CAD build for the part. Positions are in the model's coordinates, mm. Face numbers are marked on the shaded views. A direction names the side the tool comes from. Round coordinates to 2 decimals unless told otherwise and drop trailing zeros. Loops run counter-clockwise (first coordinate to the right, second up) from the corner with the lowest first, then second, coordinate; pieces in that order, holes last. Notation, with made-up numbers: M 41.25,-35.75 L 77.25,-35.75 A22 ccw 77.25,-10.75 Z; hole C 29,50 d2. An arc over 180 degrees is marked long. One line per item, written item: value. Start each with the question number.
from build123d import *

# Parameters (mm, degrees)
SKETCH2_R           = 5
BOSS_EXTRUDE1_DEPTH = 62.5
SKETCH3_R           = 8
BOSS_EXTRUDE2_DEPTH = 7.5
FILLET1_R           = 5
SKETCH4_R           = 10
BOSS_EXTRUDE3_DEPTH = 7.5
CHAMFER1_SIZE       = 2


# Some blends are built 0.0001 mm under size
with BuildPart() as part:
    # Sketch2 → Boss-Extrude1 (new, symmetric)
    with BuildSketch(Plane(origin=(0, 0, 0), x_dir=(0, 0, -1), z_dir=(1, 0, 0))):
        Circle(SKETCH2_R)
    extrude(amount=BOSS_EXTRUDE1_DEPTH, both=True)

    # Sketch3 → Boss-Extrude2 (add, symmetric)
    with BuildSketch(Plane(origin=(0, 0, 0), x_dir=(0, 0, -1), z_dir=(1, 0, 0))):
        Circle(SKETCH3_R)
    extrude(amount=BOSS_EXTRUDE2_DEPTH, both=True)

    # Fillet1
    # the kernel refuses this fillet: 5 mm, written as the material it adds along each edge
    with BuildSketch(Plane(origin=(-7.5, 0, 0), x_dir=(0, 0, -1), z_dir=(0, -1, 0))) as fillet1_piece_1:
        with BuildLine():
            CenterArc((10, -4.582575695), FILLET1_R, 113.578178478, 66.421821522)
            Line((8, 0), (7.96, 0.091651514))
            ThreePointArc((7.96, 0.091651514), (6.5, 0.1), (5, 0.1))
            Line((5, 0.1), (4.9, 0))
            Line((4.9, 0), (4.9, -4.582575695))
            Line((4.9, -4.582575695), (5, -4.582575695))
        make_face()
    revolve(axis=Axis((-7.5, 0, 0), (1, 0, 0)))
    with BuildSketch(Plane(origin=(7.5, 0, 0), x_dir=(0, 0, -1), z_dir=(0, -1, 0))) as fillet1_piece_2:
        with BuildLine():
            CenterArc((10, 4.582575695), FILLET1_R, 180, 66.421821522)
            Line((5, 4.582575695), (4.9, 4.582575695))
            Line((4.9, 4.582575695), (4.9, 0))
            Line((4.9, 0), (5, -0.1))
            ThreePointArc((5, -0.1), (6.5, -0.1), (7.96, -0.091651514))
            Line((7.96, -0.091651514), (8, 0))
        make_face()
    revolve(axis=Axis((7.5, 0, 0), (1, 0, 0)))

    # Sketch4 → Boss-Extrude3 (add, symmetric)
    with BuildSketch(Plane(origin=(0, 0, 0), x_dir=(0, 0, -1), z_dir=(1, 0, 0))):
        Circle(SKETCH4_R)
    extrude(amount=BOSS_EXTRUDE3_DEPTH, both=True)

    # Chamfer1
    chamfer1_edges = [part.edges().sort_by_distance(p)[0] for p in [
        (-7.5, 0, 10),
        (7.5, 0, 10),
    ]]
    chamfer(chamfer1_edges, length=CHAMFER1_SIZE - 0.0001)  # a hair under: the kernel refuses the full size


solid = part.part
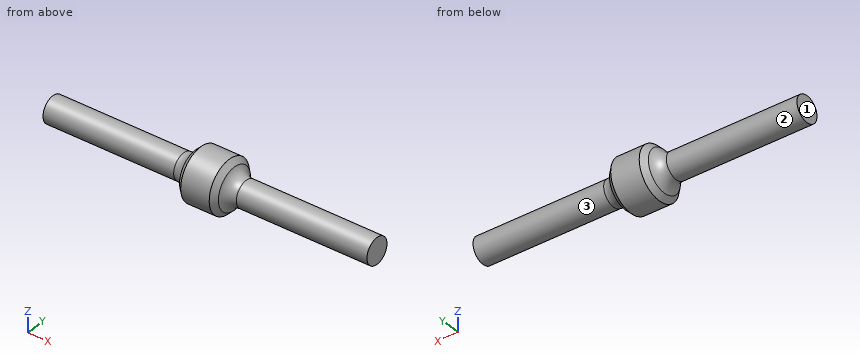
(1) Slice it at C-C, the plane x = 16.5. List the corners of the cut face in (y, z).
(2) Probe L1, parallel to Z at x = 14, y = -0.25; L2, parallel to X at y = -4.25, z = 5.75; L3, parallel to Y at x = -1.5, z = 8.75. List the from-to ranges inside material, lowest first.
(3) Flat gauge pins, fed straight in: P1, Ø8, axis at x = 29, z = 6.5, coming from the -Y side; P2, Ø1.5, axis at x = 41.5, y = 6.5, coming from the +Z side; P3, Ø5, axis at x = 35.5, z = -6, coming from the -Y side; P4, Ø10, axis at x = -32, y = -4, coming from the +Z side. Where does each tip first touch, or does it go through?
(4) Which spindle directions (+Z, -Z, +X, -X, +Y, -Y) get a long thin tool onto all of the face, cutting with end or side? Do the marked faces 1, 2 and 3. Say none if no direction does.
Check result:
1. outline: C 0,0 d10
2. L1: z = -4.99 to 4.99
2. L2: x = -7.97 to 7.97
2. L3: y = -4.84 to 4.84
3. P1: stops at y = -4.33
3. P2: passes through
3. P3: stops at y = -3.57
3. P4: stops at z = 5
4. face 1: +Z, -Z, -X, +Y, -Y
4. face 2: -X
4. face 3: +X
